Autodesk Inventor part; units mm, degrees
ref_plane "YZ Plane" through (0, 0, 0) normal (1, 0, 0) x (0, 1, 0)
ref_plane "XZ Plane" through (0, 0, 0) normal (0, 1, 0) x (-1, 0, 0)
ref_plane "XY Plane" through (0, 0, 0) normal (0, 0, 1) x (1, 0, 0)
sketch "Sketch2" plane through (0, 0, 0) normal (0, 0, 1) x (1, 0, 0)
  circle A0 centre (0, 0) radius 327.5 construction
  line L0 (-20, 307.5) -> (20, 307.5)
  line L1 (20, 307.5) -> (20, 347.5)
  line L2 (20, 347.5) -> (-20, 347.5)
  line L3 (-20, 347.5) -> (-20, 307.5)
  line L4 (-20, 307.5) -> (20, 347.5) construction
  line L5 (20, 307.5) -> (-20, 347.5) construction
  circle A1 centre (0, 327.5) radius 3.4
  circle A2 centre (-327.5, 0) radius 3.4
  line L6 (-347.5, 20) -> (-347.5, -20)
  line L7 (-347.5, -20) -> (-307.5, -20)
  line L8 (-307.5, -20) -> (-307.5, 20)
  line L9 (-307.5, 20) -> (-347.5, 20)
  line L10 (-307.5, 20) -> (-347.5, -20) construction
  line L11 (-307.5, -20) -> (-347.5, 20) construction
  circle A3 centre (0, -327.5) radius 3.4
  line L12 (-20, -347.5) -> (20, -347.5)
  line L13 (20, -347.5) -> (20, -307.5)
  line L14 (20, -307.5) -> (-20, -307.5)
  line L15 (-20, -307.5) -> (-20, -347.5)
  line L16 (-20, -307.5) -> (20, -347.5) construction
  line L17 (20, -307.5) -> (-20, -347.5) construction
  circle A4 centre (327.5, 0) radius 3.4
  line L18 (347.5, -20) -> (347.5, 20)
  line L19 (347.5, 20) -> (307.5, 20)
  line L20 (307.5, 20) -> (307.5, -20)
  line L21 (307.5, -20) -> (347.5, -20)
  line L22 (307.5, -20) -> (347.5, 20) construction
  line L23 (307.5, 20) -> (347.5, -20) construction
  line L24 (-20, 307.5) -> (-307.5, 20)
  line L25 (20, 307.5) -> (307.5, 20)
  line L26 (307.5, -20) -> (20, -307.5)
  line L27 (-20, -307.5) -> (-307.5, -20)
  line L28 (-307.5, 20) -> (307.5, 20)
  line L29 (-307.5, -20) -> (307.5, -20)
  line L30 (-20, 307.5) -> (-20, -307.5)
  line L31 (20, 307.5) -> (20, -307.5)
  line L32 (-299.2157, -28.2843) -> (28.2843, 299.2157)
  line L33 (-28.2843, 299.2157) -> (299.2157, -28.2843)
  line L34 (299.2157, 28.2843) -> (-28.2843, -299.2157)
  line L35 (-299.2157, 28.2843) -> (28.2843, -299.2157)
  line L36 (260.6, 21.1) -> (302.8, 21.1) construction
  line L37 (302.8, 21.1) -> (302.8, -21.1) construction
  line L38 (302.8, -21.1) -> (260.6, -21.1) construction
  line L39 (260.6, -21.1) -> (260.6, 21.1) construction
  line L40 (260.6, 21.1) -> (302.8, -21.1) construction
  line L41 (302.8, 21.1) -> (260.6, -21.1) construction
  circle A5 centre (297.2, 15.5) radius 1.6
  circle A6 centre (266.2, 15.5) radius 1.6
  circle A7 centre (266.2, -15.5) radius 1.6
  circle A8 centre (297.2, -15.5) radius 1.6
  circle A9 centre (-15.5, 266.2) radius 1.6
  circle A10 centre (-15.5, 297.2) radius 1.6
  circle A11 centre (15.5, 297.2) radius 1.6
  circle A12 centre (15.5, 266.2) radius 1.6
  circle A13 centre (-266.2, -15.5) radius 1.6
  circle A14 centre (-297.2, -15.5) radius 1.6
  circle A15 centre (-297.2, 15.5) radius 1.6
  circle A16 centre (-266.2, 15.5) radius 1.6
  circle A17 centre (15.5, -266.2) radius 1.6
  circle A18 centre (15.5, -297.2) radius 1.6
  circle A19 centre (-15.5, -297.2) radius 1.6
  circle A20 centre (-15.5, -266.2) radius 1.6
  point P0 (-250.9315, -20)
  point P1 (-20, -250.9315)
  point P2 (-20, -20)
  point P3 (20, -250.9315)
  point P4 (250.9315, -20)
  point P5 (20, -20)
  point P6 (250.9315, 20)
  point P7 (20, 250.9315)
  point P8 (20, 20)
  point P9 (-20, 250.9315)
  point P10 (-250.9315, 20)
  point P11 (-20, 20)
  point P12 (281.7, 0)
  dimension "d26" = 655
  dimension "d28" = 40
  dimension "d29" = 40
  dimension "d30" = 6.8
  dimension "d33" = 360
  dimension "d37" = 40
  dimension "d38" = 40
  dimension "d39" = 40
  dimension "d40" = 40
  dimension "d46" = 42.2
  dimension "d47" = 42.2
  dimension "d48" = 4.7
  dimension "d49" = 3.2
  dimension "d50" = 5.6
  dimension "d102" = 360
  dimension "d106" = 360
extrude "Extrusion3" add sketch "Sketch2" against normal blind 10 contours L3 L2 L1 L0 | L30 L33 L24 | L0 L31 L32 L33 L30 | L25 L32 L31 | L33 L30 L32 L28 L35 L24 | L33 L32 L30 | L25 L34 L28 L33 L31 L32 | L31 L33 L32 | L35 L28 L24 | L32 L33 L31 L28 L30 | L30 L28 L32 | L25 L28 L34 | L33 L28 L31 | L28 L35 L32 L29 L8 | L8 L7 L6 L9 | L28 L32 L35 | L30 L29 L35 L32 L28 | L28 L31 L29 L30 | L19 L18 L21 L20 | L20 L29 L33 L34 L28 | L34 L33 L28 | L28 L33 L34 L29 L31 | L29 L32 L27 | L35 L29 L32 | L30 L35 L29 | L29 L31 L34 L35 L30 | L26 L33 L29 | L33 L29 L34 | L29 L34 L31 | L32 L29 L35 L30 L34 L27 | L35 L34 L30 | L26 L35 L31 L34 L29 L33 | L31 L35 L34 | L34 L30 L27 | L34 L35 L31 L14 L30 | L26 L31 L35 | L14 L13 L12 L15 | A5 | A6 | A7 | A8 | A9 | A10 | A11 | A12 | A13 | A14 | A15 | A16 | A17 | A18 | A19 | A20
fillet "Fillet5" radius 4 16 edges at (-307.5, 20, -5) (-347.5, 20, -5) (-347.5, -20, -5) (-20, -347.5, -5) (20, -347.5, -5) (-20, -307.5, -5) (-20, 347.5, -5) (307.5, -20, -5) (347.5, -20, -5) (347.5, 20, -5) (20, 307.5, -5) (20, 347.5, -5) (307.5, 20, -5) (-20, 307.5, -5) (-307.5, -20, -5) (20, -307.5, -5)
extrude "Extrusion6" cut sketch "Sketch2" against normal blind 10 contours A5 | A6 | A7 | A8 | A9 | A10 | A11 | A12 | A13 | A14 | A15 | A16 | A17 | A18 | A19 | A20
equation "\"d26\" = ring_outer_diam + bar_width"
equation "\"d28\" = bar_width"
equation "\"d29\" = bar_width"
equation "\"d30\" = bar_hole_diam"
equation "\"d37\" = bar_width"
equation "\"d38\" = bar_width"
equation "\"d39\" = bar_width"
equation "\"d40\" = bar_width"
equation "\"d46\" = motor_width"
equation "\"d47\" = motor_width"
equation "\"d48\" = dist_motor_bar"
equation "\"d35\" = base_plate_thick"
equation "\"ring_inner_diam\" = 565"
equation "\"bar_width\" = 40"
equation "\"bar_hole_diam\" = 6.8"
equation "\"ring_outer_diam\" = 615"
equation "\"base_plate_thick\" = 10"
equation "\"motor_width\" = 42.2"
equation "\"dist_motor_bar\" = 4.7"
equation "\"motor_hole_diam\" = 3.2"
equation "\"motor_hole_edge_dist\" = 5.6"
properties part number "base_plate" material "Aluminum 6061"
Verification items for the finished model (mm, model axes). Give positions to 0.01 mm unless a question says otherwise; leave off trailing zeros. Write each loop counter-clockwise with the first axis right and the second up, starting at its lowest first coordinate (ties: lowest second). Pieces come first, ordered by that corner, then holes. Notation, with made-up numbers: M -5.75,47 L 23.25,47 A15 cw 23.25,58 Z; hole C -31,-13.5 d8. An arc over 180 degrees is marked long. Put each result on its own line as item: value. Start each with the question number.
1. Section check C-C (y = 60). Record the cut outline in (x, z), and give its area (3 significant figures).
2. Go/stop test with flat-tipped pins: pin 1 Ø5 at (y, z) = (37, -5) entering from -X; pin 2 Ø4 at (x, z) = (-24.5, -5.5) entering from +Y; pin 3 Ø1.5 at (y, z) = (-65.5, -5) entering from +X. Record where each tip stops, or that it passes through.
3. Scan lines: line 1 along Y through (x, z) = (-15.5, -6); line 2 along X through (y, z) = (266.2, -3.5); line 3 along X through (y, z) = (-297.2, -3.75). Record each from-to range of solid material in increasing order. Write a range as [from, to].
4. Section check B-B (x = -287). Record the cut outline in (y, z).
5. Section check A-A (z = -2). Give the number of separate pieces and of enclosed holes in the cut face, and give its area (3 significant figures).
Answer list:
1. outline: M -267.5,-10 L 267.5,-10 L 267.5,0 L -267.5,0 Z
1. area: 5,350 mm2
2. pin 1: x = -293
2. pin 2: y = 305
2. pin 3: x = 262.75
3. line 1: [-347.5, -298.8], [-295.6, -267.8], [-264.6, 264.6], [267.8, 295.6], [298.8, 347.5]
3. line 2: [-61.3, -17.1], [-13.9, 13.9], [17.1, 61.3]
3. line 3: [-30.3, -17.1], [-13.9, 13.9], [17.1, 30.3]
4. outline: M -40.5,-10 L 40.5,-10 L 40.5,0 L -40.5,0 Z
5. separate pieces: 1
5. enclosed holes: 20
5. area: 219,000 mm2
